Input: part model. Units: mm. Frame: model coordinates. A direction names the side the tool comes from. Give positions to 0.01 mm unless a question says otherwise; leave off trailing zeros. Order: outer loops, then holes, each group sorted by start corner. A loop starts at its lowest first (then second) coordinate and runs counter-clockwise, first axis right, second up. Notation, with made-up numbers: (22.25, 0.5) - (57.25, 0.5) arc R8 cw to (57.25, 10.5) - close; hole circle Ø2 at (12.25, 19). An arc over 180 degrees is marked (long way). Use a Markdown table: item, result.
from build123d import *

# Parameters (mm, degrees)
SKETCH_R      = 1.5
SKETCH_R_2    = 2
SKETCH_W      = 17
SKETCH_H      = 10
SKETCH_W_2    = 16
SKETCH_H_2    = 16
EXTRUDE_DEPTH = 3


with BuildPart() as part:
    # Sketch → Extrude (new body)
    with BuildSketch(Plane.XY):
        with BuildLine():
            Line((-104, -75.4), (104, -75.4))
            ThreePointArc((104, -75.4), (106.474874, -74.374874), (107.5, -71.9))
            Line((107.5, -71.9), (107.5, 71.9))
            ThreePointArc((107.5, 71.9), (106.474874, 74.374874), (104, 75.4))
            Line((104, 75.4), (-104, 75.4))
            ThreePointArc((-104, 75.4), (-106.474874, 74.374874), (-107.5, 71.9))
            Line((-107.5, 71.9), (-107.5, -71.9))
            ThreePointArc((-107.5, -71.9), (-106.474874, -74.374874), (-104, -75.4))
        make_face()
        with Locations((-93.5, 65.1)):
            Circle(SKETCH_R, mode=Mode.SUBTRACT)
        with Locations((63.5, 65.1)):
            Circle(SKETCH_R, mode=Mode.SUBTRACT)
        with Locations((-93.5, -44.3)):
            Circle(SKETCH_R, mode=Mode.SUBTRACT)
        with Locations((63.5, -44.3)):
            Circle(SKETCH_R, mode=Mode.SUBTRACT)
        with Locations((-20.17, -60)):
            Circle(SKETCH_R_2, mode=Mode.SUBTRACT)
        with Locations((8.83, -60)):
            Circle(SKETCH_R_2, mode=Mode.SUBTRACT)
        with Locations((-64.67, -60)):
            Circle(SKETCH_R_2, mode=Mode.SUBTRACT)
        with Locations((-36.67, -60)):
            Circle(SKETCH_R_2, mode=Mode.SUBTRACT)
        with Locations((24.83, -60)):
            Circle(SKETCH_R_2, mode=Mode.SUBTRACT)
        with Locations((53.83, -60)):
            Circle(SKETCH_R_2, mode=Mode.SUBTRACT)
        with BuildLine():
            Line((-97.5, -39.6), (67.5, -39.6))
            Line((67.5, -39.6), (71.94, -39.6))
            ThreePointArc((71.94, -39.6), (89.61767, -32.27767), (96.94, -14.6))
            Line((96.94, 35.4), (96.94, -14.6))
            ThreePointArc((96.94, 35.4), (89.61767, 53.07767), (71.94, 60.4))
            Line((67.5, 60.4), (71.94, 60.4))
            Line((67.5, 60.4), (-97.5, 60.4))
            Line((-97.5, 60.4), (-97.5, -39.6))
        make_face(mode=Mode.SUBTRACT)
        with BuildLine():
            ThreePointArc((-76.708343, -66.5), (-80.45, -52.5), (-84.191657, -66.5))
            Line((-84.191657, -66.5), (-76.708343, -66.5))
        make_face(mode=Mode.SUBTRACT)
        with Locations((-5.67, -60)):
            Rectangle(SKETCH_W, SKETCH_H, mode=Mode.SUBTRACT)
        with Locations((-50.67, -60)):
            Rectangle(SKETCH_W_2, SKETCH_H_2, mode=Mode.SUBTRACT)
        with Locations((39.33, -60)):
            Rectangle(SKETCH_W, SKETCH_H, mode=Mode.SUBTRACT)
    extrude(amount=EXTRUDE_DEPTH)


solid = part.part
1. Mould query, pull axis Y, two halves, no side actions, for faces 1 (the face through (-1, -44, 0)), 2 (the face through (53.57, -58.017, 1.479)). Classes: pulls with the +Y half, pulls with the -Y half, needs draft (parallel to the pull), parting line crosses it, or undercut.
Response:
| item | result |
|---|---|
| face 1 | needs draft |
| face 2 | undercut |
2. Section query A-A (x = 18). Return loops of the section in (y, z), then the cut area to 3 significant figures.
Response:
| item | result |
|---|---|
| outline | (-75.4, 0) - (-39.6, 0) - (-39.6, 3) - (-75.4, 3) - close; (60.4, 0) - (75.4, 0) - (75.4, 3) - (60.4, 3) - close |
| area | 152 mm^2 |
3. Set-up query: faces 3 (the face through (-1, -44, 3)), 4 (the face through (89.811, 52.882, 1.479)). Return all of +Z, -Z, +X, -X, +Y, -Y with unobstructed straight access to the full face (end or side cutting, diameter ignored); none if empty.
Response:
| item | result |
|---|---|
| face 3 | +Z, +X, -X, +Y, -Y |
| face 4 | +Z, -Z |
4. Section query D-D (z = 0.95). State how many separate pieces and enclosed holes the cut face has, then the cut area to 3 significant figures.
Response:
| item | result |
|---|---|
| separate pieces | 1 |
| enclosed holes | 15 |
| area | 12,400 mm^2 |
5. Material intervals for line 1 along Y through (x, z) = (44, 0.1); line 2 along X through (y, z) = (65.1, 2.2); line 3 along Y through (x, z) = (53.5, 1.35), sorted ascending.
Response:
| item | result |
|---|---|
| line 1 | y = -75.4 to -65, -55 to -39.6, 60.4 to 75.4 |
| line 2 | x = -107.5 to -95, -92 to 62, 65 to 107.5 |
| line 3 | y = -75.4 to -61.97, -58.03 to -39.6, 60.4 to 75.4 |
6. Section query B-B (y = 0). Return loops of the section in (x, z).
Response:
| item | result |
|---|---|
| outline | (-107.5, 0) - (-97.5, 0) - (-97.5, 3) - (-107.5, 3) - close; (96.94, 0) - (107.5, 0) - (107.5, 3) - (96.94, 3) - close |
7. Section query C-C (x = -80.45). Return loops of the section in (y, z), then the cut area to 3 significant figures.
Response:
| item | result |
|---|---|
| outline | (-75.4, 0) - (-66.5, 0) - (-66.5, 3) - (-75.4, 3) - close; (-52.5, 0) - (-39.6, 0) - (-39.6, 3) - (-52.5, 3) - close; (60.4, 0) - (75.4, 0) - (75.4, 3) - (60.4, 3) - close |
| area | 110 mm^2 |
